Verification items for the finished model (mm, model axes). Face numbers are marked on the shaded views. A direction names the side the tool comes from. Round coordinates to 2 decimals unless told otherwise and drop trailing zeros. Write each loop counter-clockwise with the first axis right and the second up, starting at its lowest first coordinate (ties: lowest second). Pieces come first, ordered by that corner, then holes. Notation, with made-up numbers: (-17, -14.75) - (37, -14.75) arc R7 cw to (37, -1.75) - close; hole circle Ø8 at (-26.5, -31.75). An arc over 180 degrees is marked (long way). Answer as a JSON object with one key per item and string values.
```python
from build123d import *

# Parameters (mm, degrees)
SKETCH1_R           = 10
BOSS_EXTRUDE1_DEPTH = 5.2
CUT_EXTRUDE1_START  = -3.4
SKETCH2_R           = 10
SKETCH2_R_2         = 4.65
CUT_EXTRUDE1_DEPTH  = 3.4
CUT_EXTRUDE2_REACH  = 16.545
SKETCH3_R           = 1.5
SKETCH4_R           = 2.95
CUT_EXTRUDE3_DEPTH  = 3.4


with BuildPart() as part:
    # Sketch1 → Boss-Extrude1 (new body)
    with BuildSketch(Plane(origin=(0, 0, 0), x_dir=(1, 0, 0), z_dir=(0, 1, 0))):
        with Locations(Location((0, 0, 0), (0, 0, 270))):
            Circle(SKETCH1_R)
    extrude(amount=BOSS_EXTRUDE1_DEPTH)

    # Sketch2 → Cut-Extrude1 (cut)
    with BuildSketch(Plane(origin=(0, 5.2, 0), x_dir=(1, 0, 0), z_dir=(0, 1, 0)).offset(CUT_EXTRUDE1_START)):
        with Locations(Location((0, 0, 0), (0, 0, 270))):
            Circle(SKETCH2_R)
        with Locations(Location((0, 0, 0), (0, 0, 270))):
            Circle(SKETCH2_R_2, mode=Mode.SUBTRACT)
    extrude(amount=CUT_EXTRUDE1_DEPTH, mode=Mode.SUBTRACT)

    # Sketch3 → Cut-Extrude2 (cut, up to next)
    with BuildSketch(Plane(origin=(0, 1.8, 0), x_dir=(1, 0, 0), z_dir=(0, 1, 0)), mode=Mode.PRIVATE) as cut_extrude2_sk1:
        with Locations(Location((0, 0, 0), (0, 0, 270))):
            Circle(SKETCH3_R)
    cut_extrude2_tool1 = extrude(cut_extrude2_sk1.sketch, amount=-CUT_EXTRUDE2_REACH, mode=Mode.PRIVATE) & part.part
    # Sketch3 → Cut-Extrude2 (cut, up to next)
    with BuildSketch(Plane(origin=(0, 1.8, 0), x_dir=(1, 0, 0), z_dir=(0, 1, 0)), mode=Mode.PRIVATE) as cut_extrude2_sk2:
        with Locations(Location((-7.5, 0, 0), (0, 0, 270))):
            Circle(SKETCH3_R)
    cut_extrude2_tool2 = extrude(cut_extrude2_sk2.sketch, amount=-CUT_EXTRUDE2_REACH, mode=Mode.PRIVATE) & part.part
    # Sketch3 → Cut-Extrude2 (cut, up to next)
    with BuildSketch(Plane(origin=(0, 1.8, 0), x_dir=(1, 0, 0), z_dir=(0, 1, 0)), mode=Mode.PRIVATE) as cut_extrude2_sk3:
        with Locations(Location((0, 7.5, 0), (0, 0, 270))):
            Circle(SKETCH3_R)
    cut_extrude2_tool3 = extrude(cut_extrude2_sk3.sketch, amount=-CUT_EXTRUDE2_REACH, mode=Mode.PRIVATE) & part.part
    # Sketch3 → Cut-Extrude2 (cut, up to next)
    with BuildSketch(Plane(origin=(0, 1.8, 0), x_dir=(1, 0, 0), z_dir=(0, 1, 0)), mode=Mode.PRIVATE) as cut_extrude2_sk4:
        with Locations(Location((7.5, 0, 0), (0, 0, 270))):
            Circle(SKETCH3_R)
    cut_extrude2_tool4 = extrude(cut_extrude2_sk4.sketch, amount=-CUT_EXTRUDE2_REACH, mode=Mode.PRIVATE) & part.part
    # Sketch3 → Cut-Extrude2 (cut, up to next)
    with BuildSketch(Plane(origin=(0, 1.8, 0), x_dir=(1, 0, 0), z_dir=(0, 1, 0)), mode=Mode.PRIVATE) as cut_extrude2_sk5:
        with Locations(Location((0, -7.5, 0), (0, 0, 270))):
            Circle(SKETCH3_R)
    cut_extrude2_tool5 = extrude(cut_extrude2_sk5.sketch, amount=-CUT_EXTRUDE2_REACH, mode=Mode.PRIVATE) & part.part
    add(cut_extrude2_tool1.solids().sort_by_distance((0, 1.8, 0))[0], mode=Mode.SUBTRACT)
    add(cut_extrude2_tool2.solids().sort_by_distance((-7.5, 1.8, 0))[0], mode=Mode.SUBTRACT)
    add(cut_extrude2_tool3.solids().sort_by_distance((0, 1.8, -7.5))[0], mode=Mode.SUBTRACT)
    add(cut_extrude2_tool4.solids().sort_by_distance((7.5, 1.8, 0))[0], mode=Mode.SUBTRACT)
    add(cut_extrude2_tool5.solids().sort_by_distance((0, 1.8, 7.5))[0], mode=Mode.SUBTRACT)

    # Sketch4 → Cut-Extrude3 (cut)
    with BuildSketch(Plane(origin=(0, 5.2, 0), x_dir=(1, 0, 0), z_dir=(0, 1, 0))):
        with Locations(Location((0, 0, 0), (0, 0, 270))):
            Circle(SKETCH4_R)
    extrude(amount=-CUT_EXTRUDE3_DEPTH, mode=Mode.SUBTRACT)


solid = part.part
```
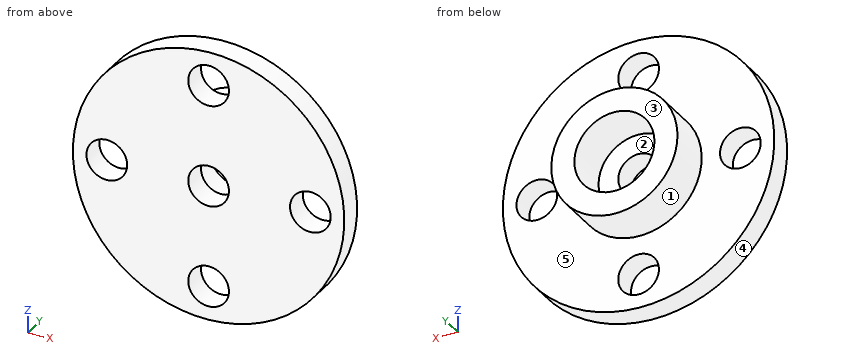
1. Cross-section at A-A (z = 0). Record the boundary of the cut face in (x, y), plus the area to 3 significant figures.
Completed:
{"outline": "(-10, 0) - (-9, 0) - (-9, 1.8) - (-10, 1.8) - close; (-6, 0) - (-1.5, 0) - (-1.5, 1.8) - (-2.95, 1.8) - (-2.95, 5.2) - (-4.65, 5.2) - (-4.65, 1.8) - (-6, 1.8) - close; (1.5, 0) - (6, 0) - (6, 1.8) - (4.65, 1.8) - (4.65, 5.2) - (2.95, 5.2) - (2.95, 1.8) - (1.5, 1.8) - close; (9, 0) - (10, 0) - (10, 1.8) - (9, 1.8) - close", "area": "31.4 mm^2"}
2. Cross-section at D-D (z = 7.5). Record the boundary of the cut face in (x, y), plus the area to 3 significant figures.
Completed:
{"outline": "(-6.61, 0) - (-1.5, 0) - (-1.5, 1.8) - (-6.61, 1.8) - close; (1.5, 0) - (6.61, 0) - (6.61, 1.8) - (1.5, 1.8) - close", "area": "18.4 mm^2"}
3. Mould release check, pull along X, two halves, no side actions. Record for the marked faces 1, 2 and 3: released by +X, released by -X, zero draft, split by the parting line, or undercut.
Completed:
{"face 1": "split by the parting line", "face 2": "undercut", "face 3": "zero draft"}
4. Access from +Z, -Z, +X, -X, +Y, -Y to the whole of each face (thin tool, end or side, straight path). Record for the marked faces 4 and 5.
Completed:
{"face 4": "+Y, -Y", "face 5": "+Y"}
5. Go/stop test with flat-tipped pins: pin 1 (1 mm diameter, centred on y = 1.5, z = 8, fed in from +X); pin 2 (2 mm diameter, centred on x = -4.5, y = 1.5, fed in from +Z); pin 3 (4 mm diameter, centred on x = 0, z = -7.5, fed in from +Y). Record where each tip stops, or that it passes through.
Completed:
{"pin 1": "stops at x = 6.61", "pin 2": "stops at z = 9.37", "pin 3": "stops at y = 1.8"}
6. Material ranges on probe 1 along X at (y, z) = (1.2, 0); probe 2 along X at (y, z) = (2.85, 0); probe 3 along X at (y, z) = (1.3, -0.75), recorded low to high. Write a range as from..to.
Completed:
{"probe 1": "x = -10..-9, -6..-1.5, 1.5..6, 9..10", "probe 2": "x = -4.65..-2.95, 2.95..4.65", "probe 3": "x = -9.97..-8.8, -6.2..-1.3, 1.3..6.2, 8.8..9.97"}
7. Cross-section at C-C (y = 0.4). Record the boundary of the cut face in (x, z).
Completed:
{"outline": "circle Ø20 at (0, 0); hole circle Ø3 at (-7.5, 0); hole circle Ø3 at (0, -7.5); hole circle Ø3 at (0, 0); hole circle Ø3 at (0, 7.5); hole circle Ø3 at (7.5, 0)"}
8. Cross-section at B-B (x = 0). Record the boundary of the cut face in (y, z).
Completed:
{"outline": "(0, -10) - (1.8, -10) - (1.8, -9) - (0, -9) - close; (0, -6) - (1.8, -6) - (1.8, -4.65) - (5.2, -4.65) - (5.2, -2.95) - (1.8, -2.95) - (1.8, -1.5) - (0, -1.5) - close; (0, 1.5) - (1.8, 1.5) - (1.8, 2.95) - (5.2, 2.95) - (5.2, 4.65) - (1.8, 4.65) - (1.8, 6) - (0, 6) - close; (0, 9) - (1.8, 9) - (1.8, 10) - (0, 10) - close"}
